Geometry: final body of the model. Coordinates: model frame, mm. Face numbers are marked on the shaded views. A direction names the side the tool comes from. Coordinates: 2 decimals unless noted, no trailing zeros. Loops run counter-clockwise (first coordinate to the right, second up) from the corner with the lowest first, then second, coordinate; pieces in that order, holes last. Notation, with made-up numbers: (47.25, 23) - (82.25, 23) arc R33 cw to (82.25, 53) - close; hole circle Ø8 at (-9, -21.75). An arc over 180 degrees is marked (long way). Answer in a Markdown table with one row per item.
from build123d import *

# Parameters (mm, degrees)
SKETCH_1_W          = 6
SKETCH_1_H          = 15
EXTRUDE_1_DEPTH     = 7
SKETCH_2_W          = 7
SKETCH_2_H          = 24
EXTRUDE_2_DEPTH     = 10
SKETCH_3_R          = 1.6
CUT_EXTRUDE_1_DEPTH = 104.07764064
CUT_EXTRUDE_2_REACH = 105.99
SKETCH_7_R          = 2.1
FILLET_1_R          = 5


with BuildPart() as part:
    # 草图1 → 凸台-拉伸1 (new body)
    with BuildSketch(Plane(origin=(0, 0, 0), x_dir=(1, 0, 0), z_dir=(0, 1, 0))):
        Polygon((7, -43), (63, -43), (63, 0), (70, 0), (70, -75), (0, -75), (0, 0), (7, 0), align=None)
        with Locations((63, -61.5)):
            Rectangle(SKETCH_1_W, SKETCH_1_H, mode=Mode.SUBTRACT)
        with Locations((7, -61.5)):
            Rectangle(SKETCH_1_W, SKETCH_1_H, mode=Mode.SUBTRACT)
    extrude(amount=EXTRUDE_1_DEPTH)

    # 草图2 → 凸台-拉伸2 (add)
    with BuildSketch(Plane.XZ):
        with Locations((3.5, 12)):
            Rectangle(SKETCH_2_W, SKETCH_2_H)
        with Locations((66.5, 12)):
            Rectangle(SKETCH_2_W, SKETCH_2_H)
    extrude(amount=EXTRUDE_2_DEPTH)

    # 草图3 → 切除-拉伸1 (cut, through all)
    with BuildSketch(Plane(origin=(70, 0, 0), x_dir=(0, 0, -1), z_dir=(1, 0, 0))):
        with Locations((-12, -4)):
            Circle(SKETCH_3_R)
        with Locations((-19, -4)):
            Circle(SKETCH_3_R)
        with Locations((-5, -4)):
            Circle(SKETCH_3_R)
    extrude(amount=-CUT_EXTRUDE_1_DEPTH, mode=Mode.SUBTRACT)

    # 草图7 → 切除-拉伸2 (cut, up to next)
    with BuildSketch(Plane(origin=(0, 7, 0), x_dir=(1, 0, 0), z_dir=(0, 1, 0)), mode=Mode.PRIVATE) as cut_extrude_2_sk1:
        with Locations(Location((19.2, -70, 0), (0, 0, 270))):
            Circle(SKETCH_7_R)
    cut_extrude_2_tool1 = extrude(cut_extrude_2_sk1.sketch, amount=-CUT_EXTRUDE_2_REACH, mode=Mode.PRIVATE) & part.part
    # 草图7 → 切除-拉伸2 (cut, up to next)
    with BuildSketch(Plane(origin=(0, 7, 0), x_dir=(1, 0, 0), z_dir=(0, 1, 0)), mode=Mode.PRIVATE) as cut_extrude_2_sk2:
        with Locations(Location((50.8, -70, 0), (0, 0, 270))):
            Circle(SKETCH_7_R)
    cut_extrude_2_tool2 = extrude(cut_extrude_2_sk2.sketch, amount=-CUT_EXTRUDE_2_REACH, mode=Mode.PRIVATE) & part.part
    add(cut_extrude_2_tool1.solids().sort_by_distance((19.2, 7, 70))[0], mode=Mode.SUBTRACT)
    add(cut_extrude_2_tool2.solids().sort_by_distance((50.8, 7, 70))[0], mode=Mode.SUBTRACT)

    # 圆角1
    fillet_1_edges = [part.edges().sort_by_distance(p)[0] for p in [
        (70, 3.5, 75),
        (0, 3.5, 75),
        (66.5, -10, 24),
        (66.5, 0, 24),
        (66.5, -10, 0),
        (3.5, -10, 0),
        (3.5, -10, 24),
        (3.5, 0, 24),
    ]]
    fillet(fillet_1_edges, radius=FILLET_1_R - 0.0001)  # a hair under: the kernel refuses the full size


solid = part.part
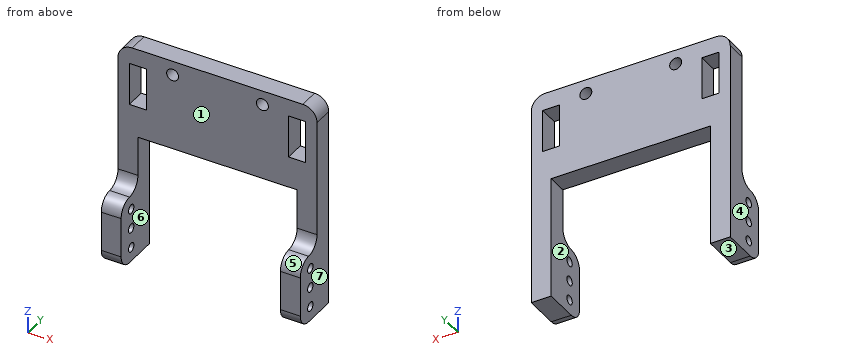
(1) Ray query, probe 1 along Y at (x, z) = (65.75, 12); probe 2 along X at (y, z) = (4.5, 16); probe 3 along Y at (x, z) = (3, 63). Return the intervals inside material, ascending.
Verdict:
| item | result |
|---|---|
| probe 1 | y = -10 to -5.6, -2.4 to 7 |
| probe 2 | x = 0 to 7, 63 to 70 |
| probe 3 | y = 0 to 7 |
(2) Cut plane D-D on z = 12. Output: boundary loops of the cut face in (x, y), then the cut area to 3 significant figures.
Verdict:
| item | result |
|---|---|
| outline | (0, -10) - (7, -10) - (7, -5.6) - (0, -5.6) - close; (0, -2.4) - (7, -2.4) - (7, 7) - (0, 7) - close; (63, -10) - (70, -10) - (70, -5.6) - (63, -5.6) - close; (63, -2.4) - (70, -2.4) - (70, 7) - (63, 7) - close |
| area | 193 mm² |
(3) Access query for the marked faces 1, 2 and 3. Directions: +Z, -Z, +X, -X, +Y, -Y. A direction counts if a zero-diameter tool reaches every point of the face in a straight line with its end or side. Return the directions, or none.
Verdict:
| item | result |
|---|---|
| face 1 | +Z, +X, -X, -Y |
| face 2 | -Z, +Y, -Y |
| face 3 | -Z, +X, -X, +Y, -Y |
(4) First-contact query: pin 1 Ø2 at (x, y) = (48.5, 2.5) entering from -Z. Flat tip, straight axial feed; report the tip coordinate or a pass-through.
Verdict:
| item | result |
|---|---|
| pin 1 | stops at z = 43 |
(5) Cut plane A-A on z = 57. Output: boundary loops of the cut face in (x, y), then the cut area to 3 significant figures.
Verdict:
| item | result |
|---|---|
| outline | (0, 0) - (4, 0) - (4, 7) - (0, 7) - close; (10, 0) - (60, 0) - (60, 7) - (10, 7) - close; (66, 0) - (70, 0) - (70, 7) - (66, 7) - close |
| area | 406 mm² |
(6) Pull-direction query (X, two-part tool) for the marked faces 4, 5, 6 and 7; classes: pulls with the +X half, pulls with the -X half, needs draft (parallel to the pull), parting line crosses it, or undercut.
Verdict:
| item | result |
|---|---|
| face 4 | pulls with the -X half |
| face 5 | needs draft |
| face 6 | undercut |
| face 7 | pulls with the +X half |
(7) Cut plane B-B on y = -6.75. Output: boundary loops of the cut face in (x, z).
Verdict:
| item | result |
|---|---|
| outline | (0, 0.32) - (7, 0.32) - (7, 23.68) - (0, 23.68) - close; (63, 0.32) - (70, 0.32) - (70, 23.68) - (63, 23.68) - close |
(8) Cut plane C-C on x = 50.8. Output: boundary loops of the cut face in (y, z).
Verdict:
| item | result |
|---|---|
| outline | (0, 43) - (7, 43) - (7, 67.9) - (0, 67.9) - close; (0, 72.1) - (7, 72.1) - (7, 75) - (0, 75) - close |
